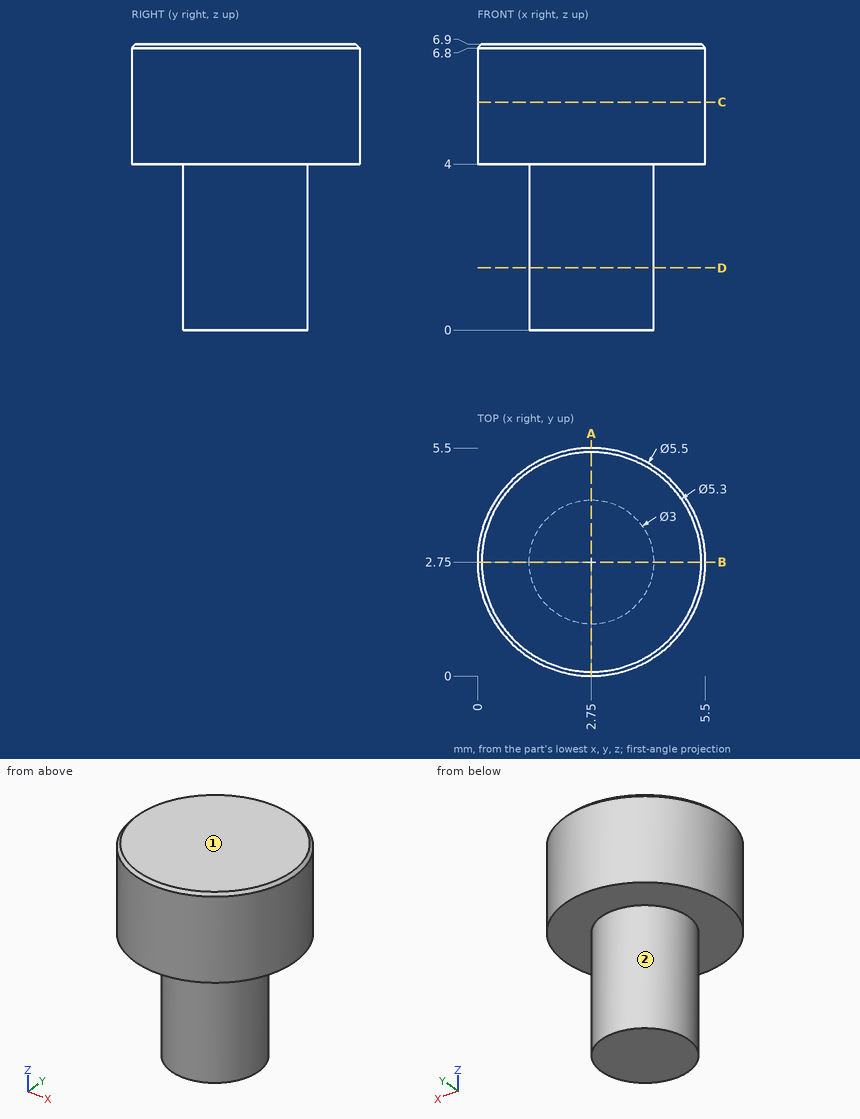
Source: three-view drawing plus pictorial views. Frame: mm from the lowest corner of the part. A direction names the side the tool comes from. Round coordinates to 2 decimals unless told otherwise and drop trailing zeros. Loops run counter-clockwise (first coordinate to the right, second up) from the corner with the lowest first, then second, coordinate; pieces in that order, holes last.
Q1. Section D-D on z = 1.5. Return loops of the section in (x, y), plus the area to 3 significant figures.
Q2. Section A-A on x = 2.75. Return loops of the section in (y, z).
Q3. Pin query (flat end, axial travel): P1, Ø1.5, axis at x = 4, z = 3.5, coming from the -Y side; P2, Ø3, axis at x = 3.5, z = 1, coming from the +Y side; P3, Ø3, axis at x = 4.5, z = 3.5, coming from the +Y side. Return the tip coordinate at first contact, or that it passes through.
Q4. Access query for the marked faces 1 and 2. Directions: +Z, -Z, +X, -X, +Y, -Y. A direction counts if a zero-diameter tool reaches every point of the face in a straight line with its end or side. Return the directions, or none.
Q5. Material intervals for L1, parallel to Z at x = 2.9, y = 4.6; L2, parallel to Y at x = 2.8, z = 1.25; L3, parallel to X at y = 2.65, z = 4.5, sorted ascending.
Q6. Section C-C on z = 5.5. Return loops of the section in (x, y), plus the area to 3 significant figures.
Evaluation:
1. outline: circle Ø3 at (2.75, 2.75)
1. area: 7.07 mm2
2. outline: (0, 4) - (1.25, 4) - (1.25, 0) - (4.25, 0) - (4.25, 4) - (5.5, 4) - (5.5, 6.8) - (5.4, 6.9) - (0.1, 6.9) - (0, 6.8) - close
3. P1: stops at y = 0.09
3. P2: stops at y = 4.25
3. P3: stops at y = 5.48
4. face 1: +Z, +X, -X, +Y, -Y
4. face 2: -Z
5. L1: z = 4 to 6.9
5. L2: y = 1.25 to 4.25
5. L3: x = 0 to 5.5
6. outline: circle Ø5.5 at (2.75, 2.75)
6. area: 23.8 mm2
